Part model, mm, in its own coordinate system. Round coordinates to 2 decimals unless told otherwise and drop trailing zeros. Order: outer loops, then holes, each group sorted by start corner. A loop starts at its lowest first (then second) coordinate and runs counter-clockwise, first axis right, second up. Notation, with made-up numbers: (85.25, 28) -> (126.25, 28) arc R27 cw to (126.25, 51) -> close; hole circle Ø9 at (-23, -22). An arc over 180 degrees is marked (long way). Answer as a JSON object with one key per item and string values. Group by question number.
```python
from build123d import *

# Parameters (mm, degrees)
BOSS_EXTRUDE1_DEPTH = 0.5953125
SKETCH2_R           = 2.7686
SKETCH2_R_2         = 1.5875
BOSS_EXTRUDE2_DEPTH = 11.1125


with BuildPart() as part:
    # Sketch1 → Boss-Extrude1 (new, symmetric)
    with BuildSketch(Plane.XY):
        Polygon((-11.1125, -20.6375), (-4.7625, 23.8125), (4.7625, 23.8125), (11.1125, -20.6375), (11.1125, -23.8125), (-11.1125, -23.8125), align=None)
    extrude(amount=BOSS_EXTRUDE1_DEPTH, both=True)

    # Sketch2 → Boss-Extrude2 (add, symmetric)
    with BuildSketch(Plane(origin=(0, 0, 0), x_dir=(0, 0, -1), z_dir=(1, 0, 0))):
        with Locations((-2.1732875, -23.8125)):
            Circle(SKETCH2_R)
        with Locations((-2.1732875, -23.8125)):
            Circle(SKETCH2_R_2, mode=Mode.SUBTRACT)
    extrude(amount=BOSS_EXTRUDE2_DEPTH, both=True)


solid = part.part
```
Q1. Band-saw the part on D-D (y = 19). List the corners of the cut face in (x, z).
Q2. Band-saw the part on B-B (z = 2.45). List the corners of the cut face in (x, y), plus the area to 3 significant figures.
Q3. Two-plate mould, pull along Y, no slides. Class faces 1 (the flat face through (0, -5, -0.595)), 2 (the cylindrical face through (-0.16, -23.83, 3.76)), 3 (the flat face through (7.893, 1.899, 0.008)): +Y half, -Y half, draft (parallel to the pull), parting line (faces both ways), or undercut.
Q4. Drop flat-ended pins along their axis: pin 1 Ø2 at (x, y) = (-2.5, -4.5) entering from +Z; pin 2 Ø1 at (x, z) = (-2, 3) entering from -Y. Give the stop position or say it passes through.
Q5. Wall check: line 1 (Z direction, x = 0, y = 10); line 2 (Y direction, x = -0.25, z = 2.5); line 3 (Y direction, x = -1, z = 2.65). Give the ranges that are in metal, low to high. Write a range as [from, to].
Completed:
{
 "1": {"outline": "(-5.45, -0.6) -> (5.45, -0.6) -> (5.45, 0.6) -> (-5.45, 0.6) -> close"},
 "2": {"outline": "(-11.11, -26.57) -> (11.11, -26.57) -> (11.11, -25.38) -> (-11.11, -25.38) -> close; (-11.11, -22.25) -> (11.11, -22.25) -> (11.11, -21.06) -> (-11.11, -21.06) -> close", "area": "53.0 mm2"},
 "3": {"face 1": "draft", "face 2": "undercut", "face 3": "+Y half"},
 "4": {"pin 1": "z = 0.6", "pin 2": "y = -26.56"},
 "5": {"line 1": "[-0.6, 0.6]", "line 2": "[-26.56, -25.37], [-22.26, -21.06]", "line 3": "[-26.54, -25.33], [-22.3, -21.09]"}
}
